Check sheet for the modelled part. Datum: model origin and axes. Units: mm. A direction names the side the tool comes from. Give positions to 0.01 mm unless a question says otherwise; leave off trailing zeros. Order: outer loops, then holes, each group sorted by start corner. A loop starts at its lowest first (then second) coordinate and runs counter-clockwise, first axis right, second up.
```python
from build123d import *

# Parameters (mm, degrees)
F1_DEPTH = 76.5
F3_DEPTH = 66
F5_W     = 8
F5_H     = 18
F6_DEPTH = 44.4045879922


with BuildPart() as f1:
    # F0 (on Top) → F1 (new body)
    with BuildSketch(Plane.XY):
        Polygon((18.8770888389, -22.3604461369), (16.375, 0), (0, 0), (-16.375, 0), (-18.8770888389, -22.3604461369), (-25.5264991533, -27.1589190681), (-25.5264991533, -33.9414753953), (-10.9456513292, -23.4193688791), (-9.5, -10.5), (0, -10.5), (9.5, -10.5), (10.9456513292, -23.4193688791), (25.5264991533, -33.9414753953), (25.5264991533, -27.1589190681), align=None)
    extrude(amount=F1_DEPTH)

    # F2 (on face) → F3 (cut)
    with BuildSketch(Plane.XY.offset(76.5)):
        Polygon((9.6, 0), (-9.6, 0), (-9.6, -3.5), (-12.9, -3.5), (-12.9, -7), (12.9, -7), (12.9, -3.5), (9.6, -3.5), align=None)
    extrude(amount=-F3_DEPTH, mode=Mode.SUBTRACT)

    # F5 (on plane+point) → F6 (cut, through all)
    with BuildSketch(Plane.YZ.offset(18.8770888389)):
        with Locations((-18.3604461369, 38.25)):
            Rectangle(F5_W, F5_H)
    extrude(amount=-F6_DEPTH, mode=Mode.SUBTRACT)


solid = f1.part
```
Q1. Material ranges on line 1 (Y direction, x = 11, z = 40.5); line 2 (Y direction, x = 1, z = 32); line 3 (X direction, y = -14.5, z = 68), recorded low to high.
Q2. Sectioned sample at C-C, the plane x = 5. Record the cut outline in (y, z).
Q3. Tool access check on faces 4 (the flat face through (-14, -14.36, 38)), 5 (the flat face through (18.134, -28.607, 37.714)), 6 (the flat face through (-12.9, -5, 44)). Record the directions out of +Z, -Z, +X, -X, +Y, -Y that give a thin tool (end or side, any length) a straight path to the whole face; none if there is none.
Q4. Sectioned sample at A-A, the plane z = 33.5. Record the cut outline in (x, y) (1 decimal), plus the area to 3 significant figures.
Q5. Go/stop test with flat-tipped pins: P1, Ø12, axis at x = -6, z = 31.5, coming from the -Y side; P2, Ø1, axis at y = -13, z = 27.5, coming from the -X side; P3, Ø1.8, axis at y = -2, z = 59, coming from the +X side. Record where each tip stops, or that it passes through.
Q6. Draft check along Z on faces 1 (the flat face through (-15, -22.36, 38)), 2 (the flat face through (-2, -9, 76.5)), 3 (the flat face through (-9.6, -2, 44)). Enter one of: pulls with the +Z half, pulls with the -Z half, needs draft (parallel to the pull), parting line crosses it, or undercut.
Q7. Sectioned sample at D-D, the plane z = 62.5. Record the cut outline in (x, y) (1 decimal).
Q8. Sectioned sample at B-B, the plane y = -25.5. Record the cut outline in (x, z).
Filled in:
1. line 1: y = -23.46 to -22.36, -14.36 to -7, -3.5 to 0
1. line 2: y = -10.5 to -7
1. line 3: x = -18 to -9.95, 9.95 to 18
2. outline: (-10.5, 0) - (0, 0) - (0, 10.5) - (-7, 10.5) - (-7, 76.5) - (-10.5, 76.5) - close
3. face 4: +X, -X
3. face 5: +Z, -Z, -Y
3. face 6: +Z
4. outline: (-25.5, -33.9) - (-10.9, -23.4) - (-10.8, -22.4) - (-18.9, -22.4) - (-25.5, -27.2) - close; (-18, -14.4) - (-9.9, -14.4) - (-9.5, -10.5) - (9.5, -10.5) - (9.9, -14.4) - (18, -14.4) - (16.4, 0) - (9.6, 0) - (9.6, -3.5) - (12.9, -3.5) - (12.9, -7) - (-12.9, -7) - (-12.9, -3.5) - (-9.6, -3.5) - (-9.6, 0) - (-16.4, 0) - close; (10.8, -22.4) - (10.9, -23.4) - (25.5, -33.9) - (25.5, -27.2) - (18.9, -22.4) - close
4. area: 413 mm2
5. P1: stops at y = -24.18
5. P2: stops at x = -17.89
5. P3: stops at x = 16.7
6. face 1: undercut
6. face 2: pulls with the +Z half
6. face 3: needs draft
7. outline: (-25.5, -33.9) - (-10.9, -23.4) - (-9.5, -10.5) - (9.5, -10.5) - (10.9, -23.4) - (25.5, -33.9) - (25.5, -27.2) - (18.9, -22.4) - (16.4, 0) - (9.6, 0) - (9.6, -3.5) - (12.9, -3.5) - (12.9, -7) - (-12.9, -7) - (-12.9, -3.5) - (-9.6, -3.5) - (-9.6, 0) - (-16.4, 0) - (-18.9, -22.4) - (-25.5, -27.2) - close
8. outline: (-23.23, 0) - (-13.83, 0) - (-13.83, 76.5) - (-23.23, 76.5) - close; (13.83, 0) - (23.23, 0) - (23.23, 76.5) - (13.83, 76.5) - close
